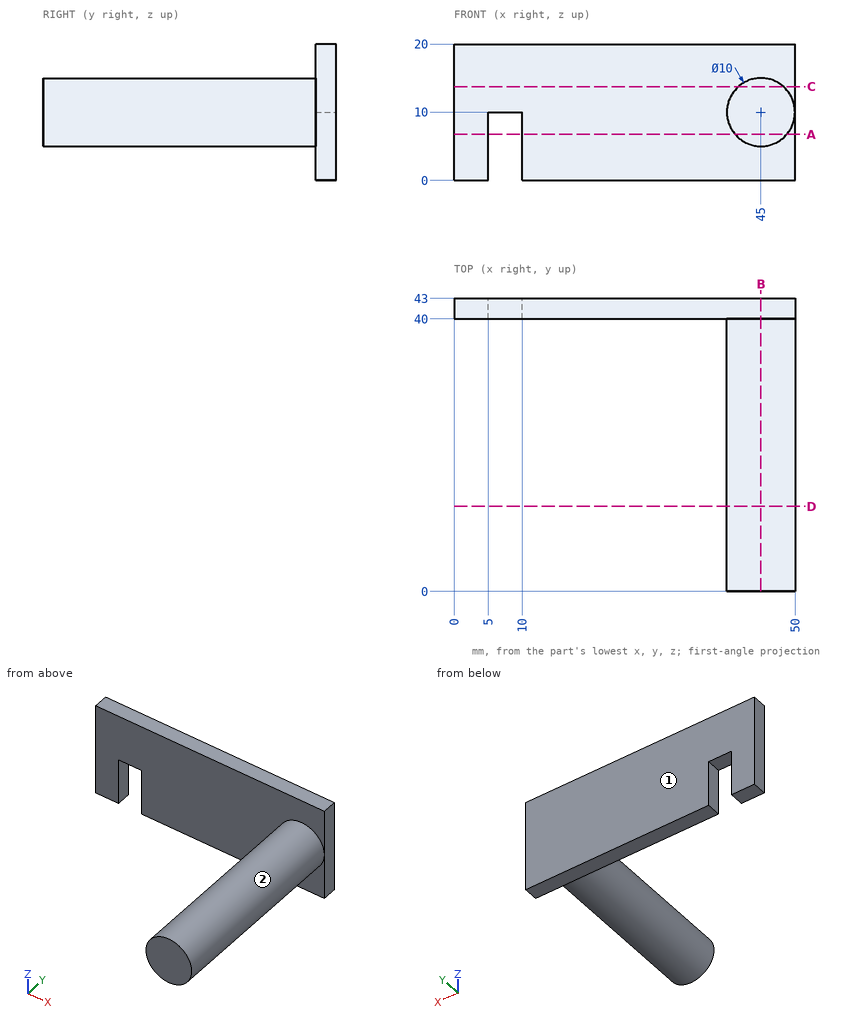
Job drawing, mm, ordinate dimensions from the low corner. One solid piece. A direction names the side the tool comes from. Coordinates: 2 decimals unless noted, no trailing zeros. Order: outer loops, then holes, each group sorted by start corner. A loop starts at its lowest first (then second) coordinate and runs counter-clockwise, first axis right, second up. Notation, with made-up numbers: (-20, -7) -> (21, -7) arc R13 ccw to (21, 4) -> close; hole circle Ø8 at (62.25, 55). An arc over 180 degrees is marked (long way). Return JSON: item names as keys, results as strings. Group by question number.
Item 1: Saw through at C-C on z = 13.75. Write the cut outline in (x, y).
Item 2: Wall check: line 1 along Y through (x, z) = (20, 3); line 2 along X through (y, z) = (28, 8.5); line 3 along X through (y, z) = (6.5, 12.75). Give the ranges that are in metal, low to high. Write a range as [from, to].
Item 3: Saw through at D-D on y = 12.5. Write the cut outline in (x, z), then the cut area to 3 significant figures.
Item 4: Saw through at B-B on x = 45. Write the cut outline in (y, z).
Item 5: Tool access for the marked faces 1 and 2: list every direction of +Z, -Z, +X, -X, +Y, -Y with a clear straight run to the whole face (end or side of a thin tool).
Item 6: Flat gauge pins, fed straight in: P1, Ø2, axis at y = 15.5, z = 13.5, coming from the +X side; P2, Ø5, axis at x = 18, z = 13.5, coming from the -Y side; P3, Ø0.9, axis at x = 8, y = 41.5, coming from the -Z side; P4, Ø0.9, axis at y = 41, z = 5, coming from the -X side. Where does each tip first touch, or does it go through?
Item 7: Saw through at A-A on z = 6.75. Write the cut outline in (x, y).
Values found:
{
 "1": {"outline": "(0, 40) -> (41.69, 40) -> (41.69, 0) -> (48.31, 0) -> (48.31, 40) -> (50, 40) -> (50, 43) -> (0, 43) -> close"},
 "2": {"line 1": "y = [40, 43]", "line 2": "x = [40.23, 49.77]", "line 3": "x = [40.82, 49.18]"},
 "3": {"outline": "circle Ø10 at (45, 10)", "area": "78.5 mm2"},
 "4": {"outline": "(0, 5) -> (40, 5) -> (40, 0) -> (43, 0) -> (43, 20) -> (40, 20) -> (40, 15) -> (0, 15) -> close"},
 "5": {"face 1": "+Z, -Z, +X, -X, +Y", "face 2": "-Y"},
 "6": {"P1": "stops at x = 49.33", "P2": "stops at y = 40", "P3": "stops at z = 10", "P4": "stops at x = 0"},
 "7": {"outline": "(0, 40) -> (5, 40) -> (5, 43) -> (0, 43) -> close; (10, 40) -> (41.2, 40) -> (41.2, 0) -> (48.8, 0) -> (48.8, 40) -> (50, 40) -> (50, 43) -> (10, 43) -> close"}
}
